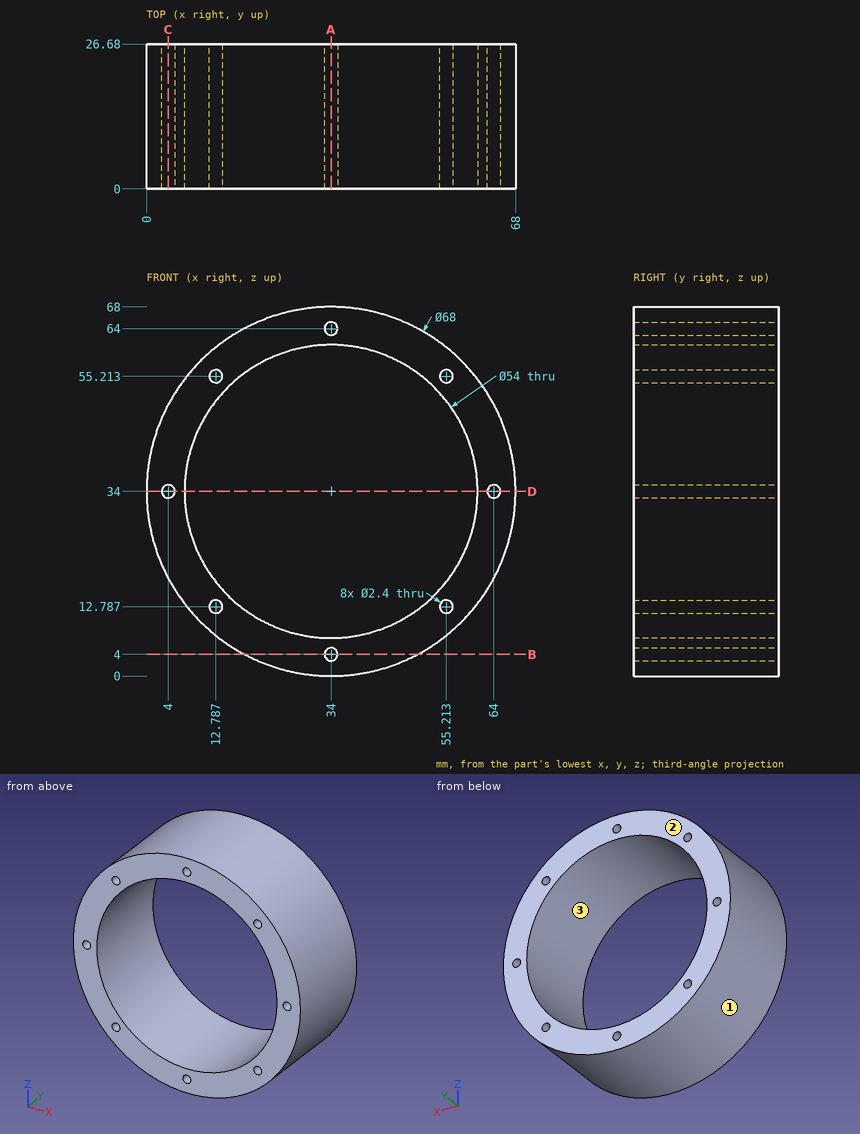
Can you work these out from the drawing? Everything is in mm from the part's minimum corner. Round coordinates to 2 decimals unless told otherwise and drop trailing zeros. Write each loop counter-clockwise with the first axis right and the second up, starting at its lowest first coordinate (ties: lowest second). Pieces come first, ordered by that corner, then holes.
1. Suppose I cut it at D-D (z = 34). List the corners of the cut face in (x, y) for me.
2. Suppose I cut it at C-C (x = 4). List the corners of the cut face in (y, z) for me.
3. If we mould it in two halves opening along X, with no side actions, what happens to the marked faces 1, 2 and 3? For each: released by +X, released by -X, zero draft, split by the parting line, or undercut.
4. Will these pins go through, and if not, where does the flat tip stop? pin 1 Ø10 at (x, y) = (14.5, 9.5) entering from -Z; pin 2 Ø6 at (y, z) = (16.5, 43) entering from -X; pin 3 Ø8 at (y, z) = (17.5, 11.5) entering from -X.
5. Suppose I cut it at A-A (x = 34). List the corners of the cut face in (y, z) for me.
6. Suppose I cut it at B-B (z = 4). List the corners of the cut face in (x, y) for me, and give its area (3 significant figures).
7. I need wall thicknesses on L1, parallel to Z at x = 34, y = 9; L2, parallel to X at y = 13.5, z = 13.5 (1 decimal); L3, parallel to X at y = 22, z = 55.5. Which ranges of each line are inside material? Lowest first, please.
Answer sheet:
1. outline: (0, 0) - (2.8, 0) - (2.8, 26.68) - (0, 26.68) - close; (5.2, 0) - (7, 0) - (7, 26.68) - (5.2, 26.68) - close; (61, 0) - (62.8, 0) - (62.8, 26.68) - (61, 26.68) - close; (65.2, 0) - (68, 0) - (68, 26.68) - (65.2, 26.68) - close
2. outline: (0, 18) - (26.68, 18) - (26.68, 32.8) - (0, 32.8) - close; (0, 35.2) - (26.68, 35.2) - (26.68, 50) - (0, 50) - close
3. face 1: split by the parting line
3. face 2: zero draft
3. face 3: undercut
4. pin 1: stops at z = 3.25
4. pin 2: stops at x = 0.53
4. pin 3: stops at x = 5.47
5. outline: (0, 0) - (26.68, 0) - (26.68, 2.8) - (0, 2.8) - close; (0, 5.2) - (26.68, 5.2) - (26.68, 7) - (0, 7) - close; (0, 61) - (26.68, 61) - (26.68, 62.8) - (0, 62.8) - close; (0, 65.2) - (26.68, 65.2) - (26.68, 68) - (0, 68) - close
6. outline: (18, 0) - (32.8, 0) - (32.8, 26.68) - (18, 26.68) - close; (35.2, 0) - (50, 0) - (50, 26.68) - (35.2, 26.68) - close
6. area: 790 mm2
7. L1: z = 0 to 2.8, 5.2 to 7, 61 to 62.8, 65.2 to 68
7. L2: x = 6.9 to 11.8, 13.8 to 16.4, 51.6 to 54.2, 56.2 to 61.1
7. L3: x = 7.66 to 11.62, 13.95 to 17.67, 50.33 to 54.05, 56.38 to 60.34
